```python
from build123d import *

# Parameters (mm, degrees)
F1_ANGLE = 180


with BuildPart() as f1:
    # F0 (on Front) → F1 (revolve)
    with BuildSketch(Plane.XZ):
        with BuildLine():
            ThreePointArc((98.9584, 1.905), (98.028464, 4.150064), (95.7834, 5.08))
            Line((95.7834, 5.08), (40.5384, 5.08))
            Line((40.5384, 5.08), (40.5384, 2.54))
            Line((40.5384, 2.54), (21.4884, 2.54))
            Line((21.4884, 2.54), (21.4884, 0))
            Line((21.4884, 0), (92.2909, 0))
            ThreePointArc((92.2909, 0), (93.413432, -0.464968), (93.8784, -1.5875))
            Line((93.8784, -1.5875), (93.8784, -23.8125))
            ThreePointArc((93.8784, -23.8125), (94.343368, -24.935032), (95.4659, -25.4))
            Line((95.4659, -25.4), (97.3709, -25.4))
            ThreePointArc((97.3709, -25.4), (98.493432, -24.935032), (98.9584, -23.8125))
            Line((98.9584, -23.8125), (98.9584, 1.905))
        make_face()
    revolve(axis=Axis((0, 0, -0.332045), (0, 0, -1)), revolution_arc=F1_ANGLE)


solid = f1.part
```
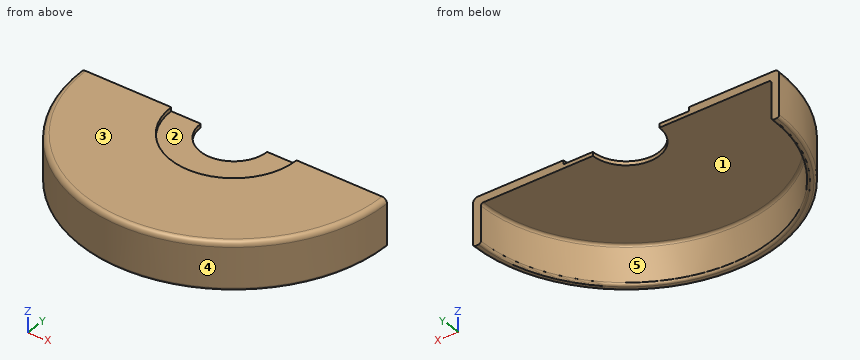
Design review of the part built by this model. Coordinates are the model's own, in mm. Face numbers are marked on the shaded views. A direction names the side the tool comes from. Coordinates: 2 decimals unless noted, no trailing zeros. Order: outer loops, then holes, each group sorted by start corner. A loop starts at its lowest first (then second) coordinate and runs counter-clockwise, first axis right, second up. Notation, with made-up numbers: M 73.25,50.25 L 125.25,50.25 A19 ccw 125.25,58.25 Z; hole C -29,-18 d7. An arc over 180 degrees is marked long. Answer as a JSON object with one key per item and string values. Group by question number.
1) For pin 1 (10 mm diameter, centred on x = 35.5, y = -75.5, fed in from -Z); pin 2 (1.5 mm diameter, centred on x = 72.5, z = -7.5, fed in from -Y); pin 3 (12 mm diameter, centred on x = 12.5, y = -22.5, fed in from +Z), all flat-tipped, find the tip position at first contact; note any pin that passes through.
2) Mouldability with a two-part tool opening along X and no side actions: class the marked faces 3, 4 and 5 as pulls with the +X half, pulls with the -X half, needs draft (parallel to the pull), parting line crosses it, or undercut.
3) Tool access review of the marked faces 1 and 2: name each direction out of +Z, -Z, +X, -X, +Y, -Y from which nothing blocks a thin tool from reaching the whole face with its end or side.
4) Wall thickness on L1, parallel to Z at x = 3.5, y = -68; L2, parallel to X at y = -60.5, z = -6.5; L3, parallel to X at y = -31.5, z = -12.5: over which ranges is each line inside the solid? List them lowest first.
5) Add section B-B, the plane z = -14. Write out the cut boundary in (x, y).
Computed values:
{
 "1": {"pin 1": "stops at z = 0", "pin 2": "stops at y = -68.15", "pin 3": "stops at z = 2.54"},
 "2": {"face 3": "needs draft", "face 4": "parting line crosses it", "face 5": "undercut"},
 "3": {"face 1": "-Z, +Y", "face 2": "+Z, +Y"},
 "4": {"L1": "z = 0 to 5.08", "L2": "x = -78.31 to -71.78, 71.78 to 78.31", "L3": "x = -93.81 to -88.44, 88.44 to 93.81"},
 "5": {"outline": "M -98.96,0 A98.96 ccw 98.96,0 L 93.88,0 A93.88 cw -93.88,0 Z"}
}
